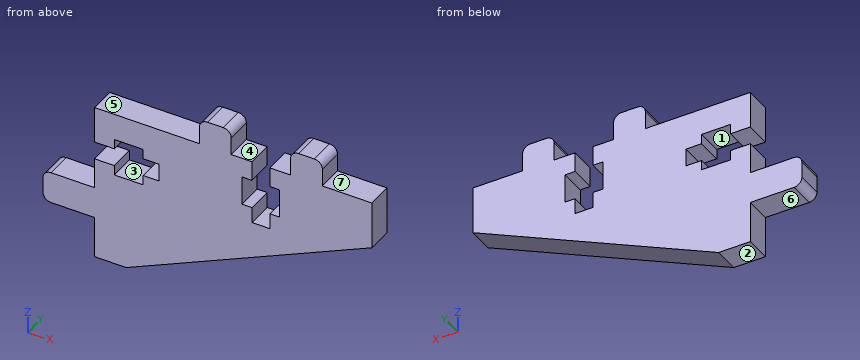
Autodesk Inventor part; units mm, degrees
ref_plane "YZ Plane" through (0, 0, 0) normal (1, 0, 0) x (0, 1, 0)
ref_plane "XZ Plane" through (0, 0, 0) normal (0, 1, 0) x (-1, 0, 0)
ref_plane "XY Plane" through (0, 0, 0) normal (0, 0, 1) x (1, 0, 0)
sketch "Sketch1" plane through (0, 0, 0) normal (0, 1, 0) x (-1, 0, 0)
  line L0 (0, -40) -> (0, 0)
  line L1 (0, 0) -> (-70, 0)
  line L2 (-70, 0) -> (-70, -12)
  line L3 (-70, -12) -> (-8, -40)
  line L4 (-8, -40) -> (0, -40)
  dimension "d0" = 8
  dimension "d1" = 12
  dimension "d2" = 70
  dimension "d3" = 40
extrude "Extrusion1" add sketch "Sketch1" along normal blind 6.5
sketch "Sketch2" plane through (0, 0, 0) normal (0, -1, 0) x (1, 0, 0)
  line L0 (0, 0) -> (0, -40)
  line L1 (70, 0) -> (0, 0)
  line L2 (39.75, 0) -> (44.25, 0)
  line L3 (44.25, -16.3) -> (39.75, -16.3)
  line L4 (46.75, -5) -> (46.75, -12.3)
  line L5 (37.25, -12.3) -> (37.25, -5)
  line L6 (37.25, -5) -> (39.75, -5)
  line L7 (44.25, -5) -> (46.75, -5)
  line L8 (46.75, -12.3) -> (44.25, -12.3)
  line L9 (39.75, -12.3) -> (37.25, -12.3)
  line L10 (39.75, -16.3) -> (39.75, -12.3)
  line L11 (39.75, -5) -> (39.75, 0)
  line L12 (44.25, 0) -> (44.25, -5)
  line L13 (44.25, -12.3) -> (44.25, -16.3)
  line L14 (0, -13.75) -> (0, -9.25)
  line L15 (16.3, -9.25) -> (16.3, -13.75)
  line L16 (5, -6.75) -> (12.3, -6.75)
  line L17 (12.3, -16.25) -> (5, -16.25)
  line L18 (5, -16.25) -> (5, -13.75)
  line L19 (5, -9.25) -> (5, -6.75)
  line L20 (12.3, -6.75) -> (12.3, -9.25)
  line L21 (12.3, -13.75) -> (12.3, -16.25)
  line L22 (16.3, -13.75) -> (12.3, -13.75)
  line L23 (5, -13.75) -> (0, -13.75)
  line L24 (0, -9.25) -> (5, -9.25)
  line L25 (12.3, -9.25) -> (16.3, -9.25)
  point P0 (42, -16.3)
  point P1 (16.3, -11.5)
  dimension "d6" = 4.5
  dimension "d7" = 4
  dimension "d8" = 5
  dimension "d9" = 7.3
  dimension "d10" = 2.5
  dimension "d11" = 4.5
  dimension "d12" = 4
  dimension "d13" = 5
  dimension "d14" = 7.3
  dimension "d15" = 2.5
  dimension "d16" = 42
  dimension "d17" = 11.5
extrude "Extrusion2" cut sketch "Sketch2" against normal through all
sketch "Sketch3" plane through (0, 0, 0) normal (0, -1, 0) x (1, 0, 0)
  line L0 (39.75, 0) -> (0, 0)
  line L1 (16.3, -9.25) -> (16.3, -13.75)
  line L2 (0, -13.75) -> (0, -40)
  line L3 (70, 0) -> (44.25, 0)
  line L4 (44.25, -16.3) -> (39.75, -16.3)
  line L5 (26.5, 0) -> (34.5, 0)
  line L6 (34.5, 0) -> (34.5, 4.5)
  line L7 (32.5, 6.5) -> (28.5, 6.5)
  line L8 (26.5, 4.5) -> (26.5, 0)
  line L9 (49.5, 0) -> (57.5, 0)
  line L10 (57.5, 0) -> (57.5, 4.5)
  line L11 (55.5, 6.5) -> (51.5, 6.5)
  line L12 (49.5, 4.5) -> (49.5, 0)
  line L13 (0, -21.5) -> (-11, -21.5)
  line L14 (-13, -23.5) -> (-13, -27.5)
  line L15 (-11, -29.5) -> (0, -29.5)
  line L16 (0, -29.5) -> (0, -21.5)
  arc A0 (28.5, 6.5) -> (26.5, 4.5) centre (28.5, 4.5) ccw
  arc A1 (34.5, 4.5) -> (32.5, 6.5) centre (32.5, 4.5) ccw
  arc A2 (51.5, 6.5) -> (49.5, 4.5) centre (51.5, 4.5) ccw
  arc A3 (57.5, 4.5) -> (55.5, 6.5) centre (55.5, 4.5) ccw
  arc A4 (-11, -21.5) -> (-13, -23.5) centre (-11, -23.5) ccw
  arc A5 (-13, -27.5) -> (-11, -29.5) centre (-11, -27.5) ccw
  point P0 (16.3, -11.5)
  point P1 (42, -16.3)
  dimension "d20" = 2
  dimension "d21" = 8
  dimension "d22" = 8
  dimension "d23" = 8
  dimension "d24" = 6.5
  dimension "d25" = 15
  dimension "d26" = 13
  dimension "d27" = 7.5
  dimension "d28" = 10
extrude "Extrusion3" add sketch "Sketch3" against normal blind 6.5
equation "\"d22\" = d21"
equation "\"d23\" = d22"
properties part number "z_axis_top_brace" material "Plywood, Finish"
Can you work these out from the model? Positions are in its coordinate system, mm. Face numbers are marked on the shaded views. A direction names the side the tool comes from. Round coordinates to 2 decimals unless told otherwise and drop trailing zeros. Loops run counter-clockwise (first coordinate to the right, second up) from the corner with the lowest first, then second, coordinate; pieces in that order, holes last.
Item 1: Suppose I cut it at A-A, the plane z = -19. Write out the boundary of the cut face in (x, y), then the cut area to 3 significant figures.
Item 2: Which directions (+Z, -Z, +X, -X, +Y, -Y) give clear straight access to the entire face, cutting with the end or side of a thin tool? Please do the marked faces 3, 4, 5, 6 and 7.
Item 3: Will these pins go through, and if not, where does the flat tip stop? pin 1 Ø3 at (y, z) = (3, -35.5) entering from -X; pin 2 Ø1.3 at (y, z) = (4, -11) entering from -X; pin 3 Ø2 at (x, y) = (40, 2.5) entering from -Z; pin 4 Ø1.5 at (x, z) = (40, -1.5) entering from +Y.
Item 4: If we mould it in two halves opening along X, with no side actions, what happens to the marked faces 1 and 2? For each: +X half, -X half, draft (parallel to the pull), parting line (faces both ways), or undercut.
Item 5: Please list where these lines run through material, in increasing order: L1, parallel to X at y = 3, z = -8; L2, parallel to Z at x = 1.5, y = 5.5; L3, parallel to Z at x = 7, y = 0.5.
Item 6: Suppose I cut it at B-B, the plane x = 53. Write out the boundary of the cut face in (y, z).
Reported:
1. outline: (0, 0) - (54.5, 0) - (54.5, 6.5) - (0, 6.5) - close
1. area: 354 mm2
2. face 3: +Y, -Y
2. face 4: +Z, +Y, -Y
2. face 5: +Z, -X, +Y, -Y
2. face 6: -Z, -X, +Y, -Y
2. face 7: +Z, +X, +Y, -Y
3. pin 1: stops at x = 0
3. pin 2: stops at x = 16.3
3. pin 3: stops at z = -26
3. pin 4: stops at y = 6.5
4. face 1: undercut
4. face 2: draft
5. L1: x = 0 to 5, 12.3 to 37.25, 46.75 to 70
5. L2: z = -40 to -13.75, -9.25 to 0
5. L3: z = -40 to -16.25, -6.75 to 0
6. outline: (0, -19.68) - (6.5, -19.68) - (6.5, 6.5) - (0, 6.5) - close
